```python
from build123d import *

# Parameters (mm, degrees)
SKETCH1_W           = 38
SKETCH1_H           = 12
BOSS_EXTRUDE1_DEPTH = 0.6
SKETCH2_W           = 26.5
SKETCH2_H           = 11.55
BOSS_EXTRUDE2_DEPTH = 1.6


with BuildPart() as part:
    # Sketch1 → Boss-Extrude1 (new, symmetric)
    with BuildSketch(Plane(origin=(0, 0, 0), x_dir=(1, 0, 0), z_dir=(0, 1, 0))):
        Rectangle(SKETCH1_W, SKETCH1_H)
    extrude(amount=BOSS_EXTRUDE1_DEPTH, both=True)

    # Sketch2 → Boss-Extrude2 (add)
    with BuildSketch(Plane.XZ.offset(0.6)):
        with Locations((-1.4, 0)):
            Rectangle(SKETCH2_W, SKETCH2_H)
    extrude(amount=BOSS_EXTRUDE2_DEPTH)


solid = part.part
```
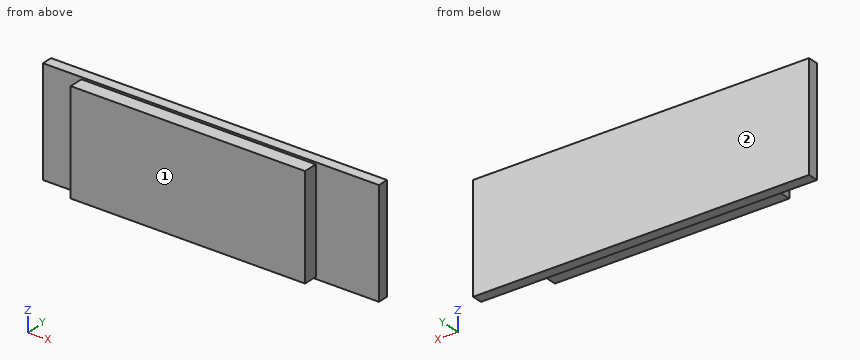
Verification items for the finished model (mm, model axes). Face numbers are marked on the shaded views. Round coordinates to 2 decimals unless told otherwise and drop trailing zeros. Write each loop counter-clockwise with the first axis right and the second up, starting at its lowest first coordinate (ties: lowest second). Pieces come first, ordered by that corner, then holes.
1. Section check B-B on z = 5. Enter the section's corners in (x, y), plus the area to 3 significant figures.
2. Section check A-A on x = 9. Enter the section's corners in (y, z) (3 decimals).
3. Draft check along Y on the marked faces 1 and 2. Enter one of: +Y half, -Y half, draft (parallel to the pull), parting line (faces both ways), or undercut.
4. Gauge pin test, flat end, axial feed: P1, Ø0.8, axis at x = -6.5, y = -1.5, coming from the +Z side (3 decimals). Record the tip position at first contact, or that the pin passes through.
5. Section check C-C on y = -1. Enter the section's corners in (x, z) (3 decimals).
6. Section check D-D on x = 15.5. Enter the section's corners in (y, z), plus the area to 3 significant figures.
7. Scan lines: L1, parallel to Y at x = 13.5, z = -4.5; L2, parallel to X at y = -0.7, z = -4.75; L3, parallel to Z at x = 7, y = -0.7 (3 decimals). Record each from-to range of solid material in increasing order.
Answer:
1. outline: (-19, -0.6) - (-14.65, -0.6) - (-14.65, -2.2) - (11.85, -2.2) - (11.85, -0.6) - (19, -0.6) - (19, 0.6) - (-19, 0.6) - close
1. area: 88.0 mm2
2. outline: (-2.2, -5.775) - (-0.6, -5.775) - (-0.6, -6) - (0.6, -6) - (0.6, 6) - (-0.6, 6) - (-0.6, 5.775) - (-2.2, 5.775) - close
3. face 1: -Y half
3. face 2: +Y half
4. P1: stops at z = 5.775
5. outline: (-14.65, -5.775) - (11.85, -5.775) - (11.85, 5.775) - (-14.65, 5.775) - close
6. outline: (-0.6, -6) - (0.6, -6) - (0.6, 6) - (-0.6, 6) - close
6. area: 14.4 mm2
7. L1: y = -0.6 to 0.6
7. L2: x = -14.65 to 11.85
7. L3: z = -5.775 to 5.775
